Design review of the part built by this model. Coordinates are the model's own, in mm. Round coordinates to 2 decimals unless told otherwise and drop trailing zeros. Loops run counter-clockwise (first coordinate to the right, second up) from the corner with the lowest first, then second, coordinate; pieces in that order, holes last. Notation, with made-up numbers: M -11,12 L 34,12 A13 ccw 34,20 Z; hole C -20,54 d8. An arc over 180 degrees is marked long. One line per item, written item: value. Start each with the question number.
Item 1: We need section B-B (y = -19). State how many separate pieces and enclosed holes the cut face has, then the cut area to 3 significant figures.
Item 2: We need section A-A (z = -3.5). Write out the cut boundary in (x, y).
Item 3: For line 1 along Y through (x, z) = (-2, -9); line 2 along X through (y, z) = (-3, -49); line 3 along X through (y, z) = (-20, -36), list the stretches that pass through material, from the lowest coordinate up.
Item 4: Clearance check with flat-ended pins moving along their axes: pin 1 (1.5 mm diameter, centred on x = 2, z = 4, fed in from +Y); pin 2 (2 mm diameter, centred on x = 2, z = 6.5, fed in from +Y); pin 3 (10 mm diameter, centred on x = 12, z = -62.5, fed in from -Y); pin 4 (5.5 mm diameter, centred on y = -17.12, z = -73.33, fed in from +X). State where each tip first meets the part, or that it passes through.
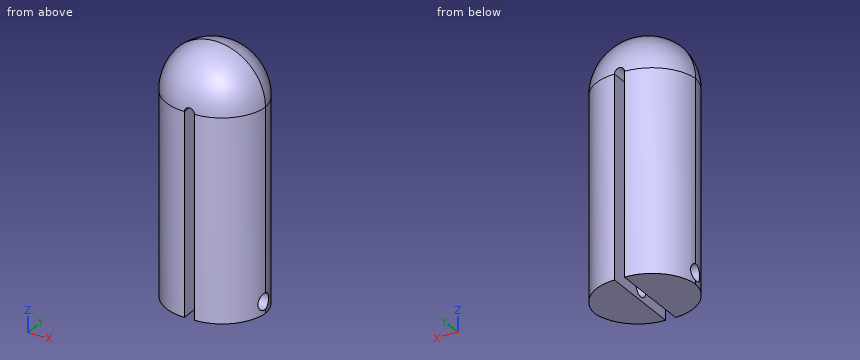
from build123d import *

# Parameters (mm, degrees)
F1_DEPTH    = 33.02
F2_T1_DEPTH = 122.514239143
F2_T3_DEPTH = 122.3049164534
F2_T6_ANGLE = 180
F2_T8_ANGLE = 180
F3_DEPTH    = 127
F5_D        = 6.35
F5_DEPTH    = 19.6628549222
F6_D        = 6.35


# Not quite as in the source:
# - a fillet or chamfer that OpenCascade refuses, or shapes differently, is made with other operations: its cross-section is extruded or revolved along the edge and cut away or added


with BuildPart() as f1:
    # F0 (on Front) → F1 (new body)
    with BuildSketch(Plane.XZ):
        with BuildLine():
            Line((-19.7072699666, 0), (19.7072699666, 0))
            ThreePointArc((19.7072699666, 0), (0, 19.7072699666), (-19.7072699666, 0))
        make_face()
        Polygon((19.7072699666, -78.064239143), (19.7072699666, 0), (-19.7072699666, 0), (-19.7072699666, -77.8549164534), align=None)
    extrude(amount=F1_DEPTH)

    # F2: fillet of radius 17.78 on 2 edges, made by hand

    # F2_s2 → F2_t1 (cut)
    with BuildSketch(Plane.XY.offset(-122.514239143)):
        with BuildLine():
            ThreePointArc((19.7072699666, -17.78), (14.4996285361, -5.2076414305), (1.9272699666, 0))
            Line((1.9272699666, 0), (19.7072699666, 0))
            Line((19.7072699666, 0), (19.7072699666, -17.78))
        make_face()
        with BuildLine():
            ThreePointArc((19.7072699666, -15.24), (14.4996285361, -27.8123585695), (1.9272699666, -33.02))
            Line((1.9272699666, -33.02), (19.7072699666, -33.02))
            Line((19.7072699666, -33.02), (19.7072699666, -15.24))
        make_face()
    extrude(amount=F2_T1_DEPTH, mode=Mode.SUBTRACT)

    # F2_s4 → F2_t3 (cut)
    with BuildSketch(Plane.XY.offset(-122.3049164534)):
        with BuildLine():
            ThreePointArc((-19.7072699666, -15.24), (-14.4996285361, -27.8123585695), (-1.9272699666, -33.02))
            Line((-1.9272699666, -33.02), (-19.7072699666, -33.02))
            Line((-19.7072699666, -33.02), (-19.7072699666, -15.24))
        make_face()
        with BuildLine():
            ThreePointArc((-19.7072699666, -17.78), (-14.4996285361, -5.2076414305), (-1.9272699666, 0))
            Line((-1.9272699666, 0), (-19.7072699666, 0))
            Line((-19.7072699666, 0), (-19.7072699666, -17.78))
        make_face()
    extrude(amount=F2_T3_DEPTH, mode=Mode.SUBTRACT)

    # F2_s5 → F2_t6 (revolve, cut)
    with BuildSketch(Plane.XY):
        with BuildLine():
            ThreePointArc((19.7072699666, -15.24), (14.4996285361, -27.8123585695), (1.9272699666, -33.02))
            Line((1.9272699666, -33.02), (19.7072699666, -33.02))
            Line((19.7072699666, -33.02), (19.7072699666, -15.24))
        make_face()
    revolve(axis=Axis((0, -33.02, 0), (0, -1, 0)), revolution_arc=F2_T6_ANGLE, mode=Mode.SUBTRACT)

    # F2_s7 → F2_t8 (revolve, cut)
    with BuildSketch(Plane.XY):
        with BuildLine():
            ThreePointArc((19.7072699666, -17.78), (14.4996285361, -5.2076414305), (1.9272699666, 0))
            Line((1.9272699666, 0), (19.7072699666, 0))
            Line((19.7072699666, 0), (19.7072699666, -17.78))
        make_face()
    revolve(axis=Axis((0, 0, 0), (0, -1, 0)), revolution_arc=F2_T8_ANGLE, mode=Mode.SUBTRACT)

    # F3 (cut): a face of the model
    f3_faces = [f1.faces().sort_by_distance(p)[0] for p in [
        (8.27376e-05, -33.02, -38.2217878295),
    ]]
    extrude(f3_faces, amount=-F3_DEPTH, mode=Mode.SUBTRACT)

    # F5 (through all, one way)
    with BuildSketch(Plane.YZ):
        with Locations((-17.1199291945, -73.3298659325)):
            Circle(F5_D / 2)
    extrude(amount=-F5_DEPTH, mode=Mode.SUBTRACT)

    # F6 (through all)
    with Locations(Plane(origin=(0, 0, 0), x_dir=(0, 1, 0), z_dir=(-1, 0, 0))):
        with Locations((-17.1199291945, 73.3298659325)):
            Hole(F6_D / 2)


solid = f1.part
A:
1. separate pieces: 3
1. enclosed holes: 0
1. area: 3,110 mm2
2. outline: M -19.66,-16.51 A17.78 ccw -1.93,-33.02 L -1.93,0 A17.78 ccw Z; M 1.93,-33.02 A17.78 ccw 19.66,-16.51 A17.78 ccw 1.93,0 Z
3. line 1: -33.02 to 0
3. line 2: -11.81 to -1.93, 1.93 to 11.81
3. line 3: -19.06 to -1.93, 1.93 to 19.06
4. pin 1: y = -0.09
4. pin 2: y = -0.43
4. pin 3: y = -32.28
4. pin 4: through
